Model file for the job. Use its own axes, mm. A direction names the side the tool comes from. Coordinates: 2 decimals unless noted, no trailing zeros. Order: outer loops, then holes, each group sorted by start corner. A loop starts at its lowest first (then second) coordinate and runs counter-clockwise, first axis right, second up.
from build123d import *

# Parameters (mm, degrees)
BOSS_EXTRUDE1_DEPTH = 1.25
BOSS_EXTRUDE5_DEPTH = 2.5
SKETCH6_W           = 5
SKETCH6_H           = 4
CUT_EXTRUDE1_DEPTH  = 1.25
CUT_EXTRUDE2_DEPTH  = 2.5


with BuildPart() as part:
    # Sketch2 → Boss-Extrude1 (new body, symmetric)
    with BuildSketch(Plane(origin=(0, 0, 0), x_dir=(1, 0, 0), z_dir=(0, 1, 0))):
        with BuildLine():
            Line((-16.109808132, 32.688266684), (-8.537351427, 60.949059844))
            ThreePointArc((-8.537351427, 60.949059844), (0, 67.5), (8.537351427, 60.949059844))
            Line((8.537351427, 60.949059844), (16.109808132, 32.688266684))
            ThreePointArc((16.109808132, 32.688266684), (18.609958913, 28.946526618), (22.871288916, 27.5))
            Line((22.871288916, 27.5), (35, 27.5))
            ThreePointArc((35, 27.5), (45.606601718, 23.106601718), (50, 12.5))
            Line((50, 12.5), (50, -12.5))
            ThreePointArc((50, -12.5), (38.284271247, -40.784271247), (10, -52.5))
            Line((10, -52.5), (-10, -52.5))
            ThreePointArc((-10, -52.5), (-38.284271247, -40.784271247), (-50, -12.5))
            Line((-50, -12.5), (-50, 12.5))
            ThreePointArc((-50, 12.5), (-45.606601718, 23.106601718), (-35, 27.5))
            Line((-35, 27.5), (-22.871288916, 27.5))
            ThreePointArc((-22.871288916, 27.5), (-18.609958913, 28.946526618), (-16.109808132, 32.688266684))
        make_face()
        with BuildLine():
            Line((6.122536861, 60.302012231), (13.694993566, 32.041219072))
            ThreePointArc((13.694993566, 32.041219072), (17.08805534, 26.963143267), (22.871288916, 25))
            Line((22.871288916, 25), (35, 25))
            ThreePointArc((35, 25), (43.838834765, 21.338834765), (47.5, 12.5))
            Line((47.5, 12.5), (47.5, -12.5))
            ThreePointArc((47.5, -12.5), (36.516504294, -39.016504294), (10, -50))
            Line((10, -50), (-10, -50))
            ThreePointArc((-10, -50), (-36.516504294, -39.016504294), (-47.5, -12.5))
            Line((-47.5, -12.5), (-47.5, 12.5))
            ThreePointArc((-47.5, 12.5), (-43.838834765, 21.338834765), (-35, 25))
            Line((-35, 25), (-22.871288916, 25))
            ThreePointArc((-22.871288916, 25), (-17.08805534, 26.963143267), (-13.694993566, 32.041219072))
            Line((-13.694993566, 32.041219072), (-6.122536861, 60.302012231))
            ThreePointArc((-6.122536861, 60.302012231), (0, 65), (6.122536861, 60.302012231))
        make_face(mode=Mode.SUBTRACT)
    extrude(amount=BOSS_EXTRUDE1_DEPTH, both=True)

    # Sketch5 → Boss-Extrude5 (add)
    with BuildSketch(Plane(origin=(0, 1.25, 0), x_dir=(1, 0, 0), z_dir=(0, 1, 0))):
        with BuildLine():
            ThreePointArc((-47.5, 12.5), (-38.661165235, 16.161165235), (-35, 25))
            ThreePointArc((-35, 25), (-43.838834765, 21.338834765), (-47.5, 12.5))
        make_face()
        with BuildLine():
            ThreePointArc((35, 25), (38.661165235, 16.161165235), (47.5, 12.5))
            ThreePointArc((47.5, 12.5), (43.838834765, 21.338834765), (35, 25))
        make_face()
        with BuildLine():
            ThreePointArc((-47.5, -12.5), (-39.791585286, -19.595919329), (-43.473512014, -29.404851181))
            ThreePointArc((-43.473512014, -29.404851181), (-46.479492188, -21.188880811), (-47.5, -12.5))
        make_face()
        with BuildLine():
            ThreePointArc((47.5, -12.5), (39.791585286, -19.595919329), (43.473512014, -29.404851181))
            ThreePointArc((43.473512014, -29.404851181), (46.479492188, -21.188880811), (47.5, -12.5))
        make_face()
    extrude(amount=-BOSS_EXTRUDE5_DEPTH)

    # Sketch6 → Cut-Extrude1 (cut)
    with BuildSketch(Plane(origin=(0, 1.25, 0), x_dir=(1, 0, 0), z_dir=(0, 1, 0))):
        with Locations((0, 66.25)):
            Rectangle(SKETCH6_W, SKETCH6_H)
        with BuildLine():
            Line((-20.493193447, 27.916333701), (-19.643873637, 25.565024308))
            ThreePointArc((-19.643873637, 25.565024308), (-17.08805534, 26.963143267), (-15.076081678, 29.070014354))
            Line((-15.076081678, 29.070014354), (-17.127452004, 30.498957945))
            ThreePointArc((-17.127452004, 30.498957945), (-18.609958913, 28.946526618), (-20.493193447, 27.916333701))
        make_face()
        with BuildLine():
            Line((20.493193447, 27.916333701), (19.643873637, 25.565024308))
            ThreePointArc((19.643873637, 25.565024308), (17.08805534, 26.963143267), (15.076081678, 29.070014354))
            Line((15.076081678, 29.070014354), (17.127452004, 30.498957945))
            ThreePointArc((17.127452004, 30.498957945), (18.609958913, 28.946526618), (20.493193447, 27.916333701))
        make_face()
        with BuildLine():
            Line((-38.284271247, -40.784271247), (-36.516504294, -39.016504294))
            ThreePointArc((-36.516504294, -39.016504294), (-34.689746158, -40.725280064), (-32.753133619, -42.308470449))
            Line((-32.753133619, -42.308470449), (-34.270009194, -44.295701812))
            ThreePointArc((-34.270009194, -44.295701812), (-36.335729235, -42.606965401), (-38.284271247, -40.784271247))
        make_face()
        with BuildLine():
            Line((34.270009194, -44.295701812), (32.753133619, -42.308470449))
            ThreePointArc((32.753133619, -42.308470449), (34.689746158, -40.725280064), (36.516504294, -39.016504294))
            Line((36.516504294, -39.016504294), (38.284271247, -40.784271247))
            ThreePointArc((38.284271247, -40.784271247), (36.335729235, -42.606965401), (34.270009194, -44.295701812))
        make_face()
        with Locations((0, -51.5)):
            Rectangle(SKETCH6_W, SKETCH6_H)
    extrude(amount=-CUT_EXTRUDE1_DEPTH, mode=Mode.SUBTRACT)

    # Sketch7 → Cut-Extrude2 (cut)
    with BuildSketch(Plane(origin=(0, 1.25, 0), x_dir=(1, 0, 0), z_dir=(0, 1, 0))):
        with BuildLine():
            ThreePointArc((-47.5, 14.791666667), (-40.281618275, 17.781618275), (-37.291666667, 25))
            ThreePointArc((-37.291666667, 25), (-43.986148678, 21.486148678), (-47.5, 14.791666667))
        make_face()
        with BuildLine():
            ThreePointArc((37.291666667, 25), (43.986148678, 21.486148678), (47.5, 14.791666667))
            ThreePointArc((47.5, 14.791666667), (40.281618275, 17.781618275), (37.291666667, 25))
        make_face()
        with BuildLine():
            ThreePointArc((-44.600502093, -27.173283714), (-42.223551432, -20.175178049), (-47.5, -15))
            ThreePointArc((-47.5, -15), (-46.479492187, -21.188880811), (-44.600502093, -27.173283714))
        make_face()
        with BuildLine():
            ThreePointArc((47.5, -15), (46.479492187, -21.188880811), (44.600502093, -27.173283714))
            ThreePointArc((44.600502093, -27.173283714), (42.223551432, -20.175178049), (47.5, -15))
        make_face()
    extrude(amount=-CUT_EXTRUDE2_DEPTH, mode=Mode.SUBTRACT)


solid = part.part
Q1. Cut at A-A, the plane z = -56.5. List the corners of the cut face in (x, y).
Established:
outline: (-9.73, -1.25) - (-7.14, -1.25) - (-7.14, 1.25) - (-9.73, 1.25) - close; (7.14, -1.25) - (9.73, -1.25) - (9.73, 1.25) - (7.14, 1.25) - close
Q2. Cut at D-D, the plane z = 22.5. List the corners of the cut face in (x, y).
Established:
outline: (-48.73, -1.25) - (-46.15, -1.25) - (-46.15, 1.25) - (-48.73, 1.25) - close; (-42.07, -1.25) - (-39.57, -1.25) - (-39.57, 1.25) - (-42.07, 1.25) - close; (39.57, -1.25) - (42.07, -1.25) - (42.07, 1.25) - (39.57, 1.25) - close; (46.15, -1.25) - (48.73, -1.25) - (48.73, 1.25) - (46.15, 1.25) - close
Q3. Cut at C-C, the plane y = 0.65. Count the separate pieces of the cut face and the enclosed holes in it, plus the area to 3 significant figures.
Established:
separate pieces: 6
enclosed holes: 4
area: 989 mm2
Q4. Which spindle directions (+Z, -Z, +X, -X, +Y, -Y) get a long thin tool onto all of the face, cutting with end or side? Do faces 5 (the face through (0, 0, -66)), 6 (the face through (-29, 0, -27.5)), 7 (the face through (10, 1.25, -48)), 8 (the face through (-29.4, 0.02, 44.59)). Say none if no direction does.
Established:
face 5: +Z, -Z, +Y
face 6: -Z, -X, +Y, -Y
face 7: +Z, -Z, +X, -X, +Y
face 8: +Y, -Y
Q5. Probe line 1 (X direction, y = 0.4, z = 27); line 2 (Z direction, x = 44, y = 0.9); line 3 (X direction, y = 0.5, z = -11.5). List the from-to ranges inside material, lowest first.
Established:
line 1: x = -47.28 to -44.67, -44.4 to -41.13, 41.13 to 44.4, 44.67 to 47.28
line 2: z = -24.5 to -21.47, -15.41 to -13, 13.78 to 16.94, 26.62 to 33.57
line 3: x = -50 to -47.5, 47.5 to 50
Q6. Cut at B-B, the plane x = -1. List the corners of the cut face in (y, z).
Established:
outline: (-1.25, -67.44) - (0, -67.44) - (0, -64.92) - (-1.25, -64.92) - close; (-1.25, 50) - (0, 50) - (0, 52.5) - (-1.25, 52.5) - close
Q7. Drop flat-ended pins along their axis: P1, Ø1.5, axis at x = 0.5, z = -66, coming from the +Y side; P2, Ø1.4, axis at y = 1, z = -66, coming from the +X side; P3, Ø1.2, axis at x = -28.5, y = 0.5, coming from the -Z side. Give the stop position or say it passes through.
Established:
P1: stops at y = 0
P2: stops at x = 5.84
P3: stops at z = -27.5
Q8. Mould opens along Z. For faces 1 (the face through (-37.972, -0.26, 41.094)), 2 (the face through (45.49, 0.02, -23.22)), 3 (the face through (0, 0, 51)), 4 (the face through (46.5, 0, 21.1)) say: pulls with the +Z half, pulls with the -Z half, needs draft (parallel to the pull), parting line crosses it, or undercut.
Established:
face 1: pulls with the +Z half
face 2: pulls with the -Z half
face 3: needs draft
face 4: undercut
